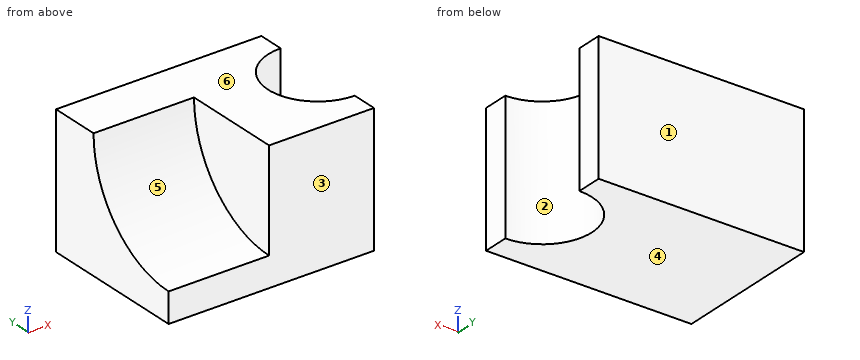
```python
from build123d import *

# Parameters (mm, degrees)
F0_W     = 103.8427650928
F0_H     = 65.8238306642
F1_DEPTH = 76.2
F3_DEPTH = 69.596
F5_DEPTH = 50.8


with BuildPart() as f1:
    # F0 (on Front) → F1 (new body)
    with BuildSketch(Plane.XZ):
        with Locations((-5.3907446563, 1.1348947883)):
            Rectangle(F0_W, F0_H)
    extrude(amount=F1_DEPTH)

    # F2 (on face) → F3 (cut)
    with BuildSketch(Plane.XY.offset(34.0468101203)):
        with BuildLine():
            Line((46.5306378901, -63.1833607248), (46.5306378901, -13.0166392752))
            ThreePointArc((46.5306378901, -13.0166392752), (21.4472771653, -38.1), (46.5306378901, -63.1833607248))
        make_face()
    extrude(amount=-F3_DEPTH, mode=Mode.SUBTRACT)

    # F4 (on face) → F5 (cut)
    with BuildSketch(Plane(origin=(-57.3121272027, 0, 0), x_dir=(0, -1, 0), z_dir=(-1, 0, 0))):
        with BuildLine():
            ThreePointArc((25.4, 34.0468101203), (40.2789755157, -1.8742143639), (76.2, -16.7531898797))
            Line((76.2, -16.7531898797), (76.2, 34.0468101203))
            Line((76.2, 34.0468101203), (25.4, 34.0468101203))
        make_face()
    extrude(amount=-F5_DEPTH, mode=Mode.SUBTRACT)


solid = f1.part
```
The listing builds one solid part. Answer for the finished solid, in the listing's coordinates (mm). Face numbers are marked on the shaded views. A direction names the side the tool comes from. Give positions to 0.01 mm unless a question says otherwise; leave off trailing zeros. Write each loop counter-clockwise with the first axis right and the second up, starting at its lowest first coordinate (ties: lowest second). Pieces come first, ordered by that corner, then holes. Notation, with made-up numbers: (-17, -16.75) -> (-2, -16.75) arc R23 cw to (-2, -4.75) -> close; hole circle Ø11 at (39.25, 58). An arc over 180 degrees is marked (long way). Write item = value, one per line. Start each with the question number.
1) Which of the six approach directions +Z, -Z, +X, -X, +Y, -Y give full straight-line access (tool end or side, diameter ignored) to the marked faces 5 and 6?
2) The part is cut by section B-B, the plane z = -26. Determine the outline of the cut face in (x, y), and give its area (3 significant figures).
3) Each of these flat-tipped pins is pushed along its axis until it touches: pin 1 (5 mm diameter, centred on x = -28, y = -61.5, fed in from +Z); pin 2 (3 mm diameter, centred on x = -27, y = -62.5, fed in from +Z); pin 3 (1.5 mm diameter, centred on y = -40, z = 19, fed in from +X). Where does it stop, or does it pass through?
4) The part is cut by section C-C, the plane y = -48.5. Determine the outline of the cut face in (x, z).
5) The part is cut by section A-A, the plane x = 33.5. Determine the outline of the cut face in (y, z).
6) The part is cut by section D-D, the plane x = -32. Determine the outline of the cut face in (y, z), and give its area (3 significant figures).
7) Straight lines are drawn through the part: line 1 along X through (y, z) = (-37, 25.5); line 2 along Y through (x, z) = (30, -25); line 3 along Y through (x, z) = (37, 19). For each, find the intervals that lie inside material, in ascending order.
8) Determine the mould class of the marked faces 1, 2, 3 and 4 for opening direction Y: +Y half, -Y half, draft (parallel to the pull), parting line (faces both ways), or undercut.
Solutions:
q1.face_5 = +Z, -X, -Y
q1.face_6 = +Z, +X, -X, +Y, -Y
q2.outline = (-57.31, -76.2) -> (46.53, -76.2) -> (46.53, -63.18) arc R25.08 cw to (46.53, -13.02) -> (46.53, 0) -> (-57.31, 0) -> close
q2.area = 6,920 mm²
q3.pin_1 = -13.75
q3.pin_2 = -14.43
q3.pin_3 = 21.59
q4.outline = (-57.31, -31.78) -> (23.7, -31.78) -> (23.7, 34.05) -> (-6.51, 34.05) -> (-6.51, -8.54) -> (-57.31, -8.54) -> close
q5.outline = (-76.2, -31.78) -> (-59.53, -31.78) -> (-59.53, 34.05) -> (-76.2, 34.05) -> close; (-16.67, -31.78) -> (0, -31.78) -> (0, 34.05) -> (-16.67, 34.05) -> close
q6.outline = (-76.2, -31.78) -> (0, -31.78) -> (0, 34.05) -> (-25.4, 34.05) arc R50.8 cw to (-76.2, -16.75) -> close
q6.area = 2,990 mm²
q7.line_1 = -6.51 to 21.47
q7.line_2 = -76.2 to -56.97, -19.23 to 0
q7.line_3 = -76.2 to -61.3, -14.9 to 0
q8.face_1 = +Y half
q8.face_2 = undercut
q8.face_3 = -Y half
q8.face_4 = draft
